Design review of the part built by this model. Coordinates are the model's own, in mm. Face numbers are marked on the shaded views. A direction names the side the tool comes from. Round coordinates to 2 decimals unless told otherwise and drop trailing zeros. Loops run counter-clockwise (first coordinate to the right, second up) from the corner with the lowest first, then second, coordinate; pieces in that order, holes last. Notation, with made-up numbers: (-35.5, -21) - (-5.5, -21) arc R8 ccw to (-5.5, -15) - close; hole circle Ø4 at (12.25, 86). An arc over 180 degrees is marked (long way). Use one line per item in the form item = value. Start each with the question number.
(1) Wall thickness on probe 1 along X at (y, z) = (2.5, -44.5); probe 2 along Z at (x, y) = (3, 1.5); probe 3 along Z at (x, y) = (12, 2): over which ranges is each line inside the solid? List them lowest first. Write a range as [from, to].
(2) We need section B-B, the plane z = -42. Write out the cut boundary in (x, y), then the cut area to 3 significant figures.
(3) For pin 1 (2 mm diameter, centred on x = 1.5, y = 2, fed in from +Z); pin 2 (1.2 mm diameter, centred on y = 2, z = -2, fed in from +X); pin 3 (1.2 mm diameter, centred on x = 1.5, y = 2, fed in from -Z), all flat-tipped, find the tip position at first contact; note any pin that passes through.
(4) We need section C-C, the plane x = 23.5. Write out the cut boundary in (y, z), then the cut area to 3 significant figures.
(5) We need section D-D, the plane y = 6.25. Write out the cut boundary in (x, z), then the cut area to 3 significant figures.
(6) Machinability: for the marked faces 1 and 2, which of the approach directions +Z, -Z, +X, -X, +Y, -Y give a long, thin tool a straight path to every point of the face, cutting with its end or side? Answer none if there is none.
(7) We need section A-A, the plane x = 42. Write out the cut boundary in (y, z).
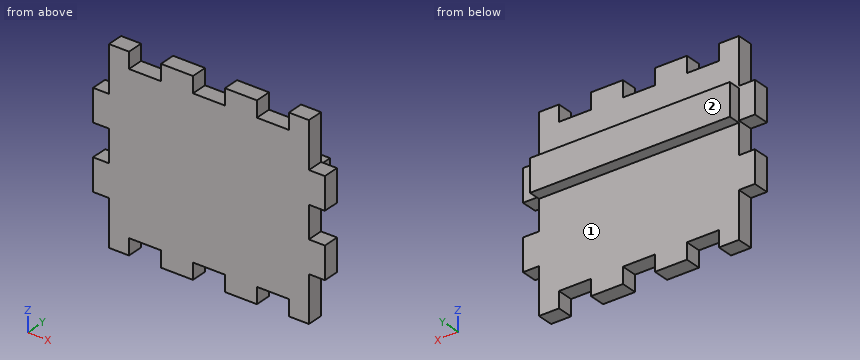
Autodesk Inventor part; units mm, degrees
ref_plane "YZ Plane" through (0, 0, 0) normal (1, 0, 0) x (0, 1, 0)
ref_plane "XZ Plane" through (0, 0, 0) normal (0, 1, 0) x (-1, 0, 0)
ref_plane "XY Plane" through (0, 0, 0) normal (0, 0, 1) x (1, 0, 0)
sketch "Sketch1" plane through (0, 0, 0) normal (0, 1, 0) x (-1, 0, 0)
  line L0 (0, 0) -> (-58, 0)
  line L1 (-58, 0) -> (-58, -47)
  line L2 (-58, -47) -> (0, -47)
  line L3 (0, -47) -> (0, 0)
  dimension "d0" = 58
  dimension "d1" = 47
extrude "Extrusion1" add sketch "Sketch1" along normal blind 4
sketch "Sketch2" plane through (0, 4, 0) normal (0, 1, 0) x (1, 0, 0)
  line L0 (58, 47) -> (0, 47)
  line L1 (0, 47) -> (0, 0)
  line L2 (0, 0) -> (58, 0)
  line L3 (58, 0) -> (58, 47)
  line L4 (4, 43) -> (54, 43)
  line L5 (54, 43) -> (54, 4)
  line L6 (54, 4) -> (4, 4)
  line L7 (4, 4) -> (4, 43)
  line L8 (4, 47) -> (4, 35.5)
  line L9 (4, 35.5) -> (0, 35.5)
  line L10 (0, 47) -> (4, 47)
  line L11 (0, 35.5) -> (0, 47)
  line L12 (0, 23.5) -> (58, 23.5) construction
  line L13 (4, 27.5) -> (0, 27.5)
  line L14 (0, 27.5) -> (0, 23.5)
  line L15 (4, 27.5) -> (4, 23.5)
  line L16 (29, 23.5) -> (29, 47) construction
  line L17 (9, 47) -> (9, 43)
  line L18 (9, 43) -> (17, 43)
  line L19 (17, 43) -> (17, 47)
  line L20 (9, 47) -> (17, 47)
  line L21 (25, 47) -> (25, 43)
  line L22 (29, 43) -> (25, 43)
  line L23 (25, 47) -> (29, 47)
  line L24 (54, 47) -> (54, 35.5)
  line L25 (54, 35.5) -> (58, 35.5)
  line L26 (58, 47) -> (54, 47)
  line L27 (58, 35.5) -> (58, 47)
  line L28 (54, 27.5) -> (58, 27.5)
  line L29 (58, 27.5) -> (58, 23.5)
  line L30 (54, 27.5) -> (54, 23.5)
  line L31 (49, 47) -> (49, 43)
  line L32 (49, 43) -> (41, 43)
  line L33 (41, 43) -> (41, 47)
  line L34 (49, 47) -> (41, 47)
  line L35 (33, 47) -> (33, 43)
  line L36 (29, 43) -> (33, 43)
  line L37 (33, 47) -> (29, 47)
  line L38 (58, 0) -> (0, 0)
  line L39 (4, 4) -> (54, 4)
  line L40 (4, 0) -> (4, 11.5)
  line L41 (4, 11.5) -> (0, 11.5)
  line L42 (0, 0) -> (4, 0)
  line L43 (0, 11.5) -> (0, 0)
  line L44 (4, 19.5) -> (0, 19.5)
  line L45 (0, 19.5) -> (0, 23.5)
  line L46 (4, 19.5) -> (4, 23.5)
  line L47 (29, 23.5) -> (29, 0) construction
  line L48 (9, 0) -> (9, 4)
  line L49 (9, 4) -> (17, 4)
  line L50 (17, 4) -> (17, 0)
  line L51 (9, 0) -> (17, 0)
  line L52 (25, 0) -> (25, 4)
  line L53 (29, 4) -> (25, 4)
  line L54 (25, 0) -> (29, 0)
  line L55 (58, 19.5) -> (58, 23.5)
  line L56 (54, 19.5) -> (54, 23.5)
  line L57 (54, 11.5) -> (58, 11.5)
  line L58 (58, 11.5) -> (58, 0)
  line L59 (58, 0) -> (54, 0)
  line L60 (29, 4) -> (33, 4)
  line L61 (33, 0) -> (33, 4)
  line L62 (33, 0) -> (29, 0)
  line L63 (54, 19.5) -> (58, 19.5)
  line L64 (54, 0) -> (54, 11.5)
  line L65 (49, 4) -> (41, 4)
  line L66 (41, 4) -> (41, 0)
  line L67 (49, 0) -> (49, 4)
  line L68 (49, 0) -> (41, 0)
  dimension "d8" = 4
  dimension "d11" = 8
  dimension "d12" = 8
  dimension "d13" = 4
  dimension "d16" = 4
  dimension "d17" = 8
extrude "Extrusion2" cut sketch "Sketch2" against normal up to surface (4 mm away) contours L3 L25 L5 L24 L0 | L31 L4 L33 L0 | L3 L63 L5 L28 | L35 L4 L21 L0 | L3 L2 L64 L5 L57 | L19 L4 L17 L0 | L2 L66 L6 L67 | L8 L7 L9 L1 L0 | L2 L52 L6 L61 | L13 L7 L44 L1 | L2 L48 L6 L50 | L41 L7 L40 L2 L1
sketch "Sketch3" plane through (0, 4, 0) normal (0, 1, 0) x (1, 0, 0)
  line L0 (4, 11.5) -> (4, 0)
  line L1 (4, 12) -> (54, 12)
  line L2 (54, 12) -> (54, 20)
  line L3 (54, 20) -> (4, 20)
  line L4 (4, 20) -> (4, 12)
  line L5 (9, 4) -> (17, 4)
  point P0 (0, 0)
  dimension "d18" = 8
  dimension "d19" = 8
extrude "Extrusion3" add sketch "Sketch3" along normal blind 3
properties part number "front" material "PBT Plastic Black"
Data:
q1.probe_1 = [4, 9], [17, 25], [33, 41], [49, 54]
q1.probe_2 = [-35.5, -27.5], [-19.5, -11.5]
q1.probe_3 = [-43, -4]
q2.outline = (4, 0) - (54, 0) - (54, 4) - (4, 4) - close
q2.area = 200 mm^2
q3.pin_1 = -11.5
q3.pin_2 = 54
q3.pin_3 = -35.5
q4.outline = (0, -47) - (4, -47) - (4, -20) - (7, -20) - (7, -12) - (4, -12) - (4, 0) - (0, 0) - close
q4.area = 212 mm^2
q5.outline = (4, -20) - (54, -20) - (54, -12) - (4, -12) - close
q5.area = 400 mm^2
q6.face_1 = -Z, +X, -X, +Y
q6.face_2 = +Z, -Z, +X, -X, +Y
q7.outline = (0, -43) - (4, -43) - (4, -20) - (7, -20) - (7, -12) - (4, -12) - (4, -4) - (0, -4) - close
